Read the model definition and answer for the solid it produces. Units are mm, in the model's axes. A direction names the side the tool comes from. Round coordinates to 2 decimals unless told otherwise and drop trailing zeros. Order: outer loops, then holes, each group sorted by start corner. A loop starts at its lowest first (then second) coordinate and runs counter-clockwise, first axis right, second up. Notation, with made-up numbers: (85, -22.5) - (95, -22.5) arc R25 cw to (95, 12.5) - close; hole circle Ø6 at (4, 31). An arc over 180 degrees is marked (long way). Answer as a JSON object with one key per item and string values. Group by question number.
Q1. Given pin 1 Ø6.5 at (x, y) = (-17.5, 6.12) entering from -Z; pin 2 Ø1.5 at (y, z) = (2, 8.5) entering from -X; pin 3 Ø10 at (x, z) = (3.5, 21.5) entering from +Y, each flat-ended and moving along its own axis, determine where each tip first touches the part or whether it passes through.
Q2. A tool of negligible diameter and unlimited length cuts with its end or side. For faces 4 (the flat face through (-20.5, 9.2, 6)), 5 (the cylindrical face through (-9.34, 0.51, 4.31)), 6 (the cylindrical face through (-20.674, 3.689, -0.084)), from which of +Z, -Z, +X, -X, +Y, -Y can it reach the whole face along a straight path? Write none if from no direction.
Q3. A cutting plane is placed at D-D on z = 23.5. Determine the outline of the cut face in (x, y).
Q4. A cutting plane is placed at B-B on y = 4. Determine the outline of the cut face in (x, z), and give its area (3 significant figures).
Q5. Consider line 1 (Z direction, x = -7.5, y = 0.2); line 2 (Z direction, x = 7.5, y = 0.35); line 3 (Y direction, x = 8, z = -10). Determine where each line is inside the solid, lowest interval first.
Q6. A cutting plane is placed at A-A on x = -17.5. Determine the outline of the cut face in (y, z).
Q7. The mould has two halves that part along Y. Classify faces 1 (the flat face through (-14, 5, 30)), 2 (the flat face through (-18, 0, 0)), 3 (the cylindrical face through (-20.674, 3.689, -24.084)): pulls with the +Y half, pulls with the -Y half, needs draft (parallel to the pull), parting line crosses it, or undercut.
Q8. A cutting plane is placed at C-C on x = 7.5. Determine the outline of the cut face in (y, z), and give its area (3 significant figures).
```python
from build123d import *

# Parameters (mm, degrees)
SKETCH1_W           = 30
SKETCH1_H           = 60
BOSS_EXTRUDE1_DEPTH = 3
SKETCH2_R           = 4
BOSS_EXTRUDE2_DEPTH = 12
SKETCH3_R           = 4
BOSS_EXTRUDE3_DEPTH = 6
SKETCH8_R           = 2.5
CUT_EXTRUDE1_DEPTH  = 4
CHAMFER1_SIZE       = 1
CHAMFER1_SIZE2      = 2
SKETCH9_R           = 4
BOSS_EXTRUDE4_DEPTH = 2


with BuildPart() as part:
    # Sketch1 → Boss-Extrude1 (new body)
    with BuildSketch(Plane(origin=(0, 0, 0), x_dir=(1, 0, 0), z_dir=(0, 1, 0))):
        Rectangle(SKETCH1_W, SKETCH1_H)
    extrude(amount=BOSS_EXTRUDE1_DEPTH)

    # Sketch2 → Boss-Extrude2 (add)
    with BuildSketch(Plane.XY.offset(30)):
        with BuildLine():
            Line((-15, 0), (-20, 0))
            ThreePointArc((-20, 0), (-17.5, 12.735742832), (-15, 0))
        make_face()
        with Locations((-17.5, 6.122498999)):
            Circle(SKETCH2_R, mode=Mode.SUBTRACT)
    boss_extrude2 = extrude(amount=-BOSS_EXTRUDE2_DEPTH)

    # Mirror1: Boss-Extrude2 across plane
    add(boss_extrude2.mirror(Plane.XY))

    # Sketch3 → Boss-Extrude3 (add, symmetric)
    with BuildSketch(Plane.XY):
        with BuildLine():
            Line((-19.72149558, 0), (-15.27850442, 0))
            ThreePointArc((-15.27850442, 0), (-17.5, 12.635565605), (-19.72149558, 0))
        make_face()
        with Locations((-17.5, 6.122498999)):
            Circle(SKETCH3_R, mode=Mode.SUBTRACT)
    extrude(amount=BOSS_EXTRUDE3_DEPTH, both=True)

    # Sketch8 → Cut-Extrude1 (cut, through all)
    with BuildSketch(Plane(origin=(0, 3, 0), x_dir=(1, 0, 0), z_dir=(0, 1, 0))):
        with Locations((7.5, -18)):
            Circle(SKETCH8_R)
        with Locations((-7.5, -6)):
            Circle(SKETCH8_R)
        with Locations((7.5, 6)):
            Circle(SKETCH8_R)
        with Locations((-7.5, 18)):
            Circle(SKETCH8_R)
    extrude(amount=-CUT_EXTRUDE1_DEPTH, mode=Mode.SUBTRACT)

    # Chamfer1
    chamfer1_edges = [part.edges().sort_by_distance(p)[0] for p in [
        (-10, 3, -18),
        (-10, 3, 6),
        (5, 3, 18),
        (5, 3, -6),
    ]]
    chamfer1_side = [part.faces().sort_by_distance(p)[0] for p in [
        (0.987193721, 3, 0),
    ]]
    chamfer(chamfer1_edges, length=CHAMFER1_SIZE, length2=CHAMFER1_SIZE2, reference=chamfer1_side[0])

    # Sketch9 → Boss-Extrude4 (add)
    with BuildSketch(Plane.XY.offset(30)):
        with Locations((-17.5, 6.122498999)):
            Circle(SKETCH9_R)
    extrude(amount=-BOSS_EXTRUDE4_DEPTH)


solid = part.part
```
Result set:
{
 "1": {"pin 1": "stops at z = 28", "pin 2": "stops at x = -15", "pin 3": "stops at y = 3"},
 "2": {"face 4": "-X, +Y", "face 5": "+Y, -Y", "face 6": "-Z"},
 "3": {"outline": "(-20, 0) - (15, 0) - (15, 3) - (-11.67, 3) arc R6.61 ccw (long way) to start; hole circle Ø8 at (-17.5, 6.12)"},
 "4": {"outline": "(-23.76, -30) - (-20.89, -30) - (-20.89, -18) - (-23.76, -18) - close; (-23.76, 18) - (-20.89, 18) - (-20.89, 28) - (-14.11, 28) - (-14.11, 18) - (-11.24, 18) - (-11.24, 30) - (-23.76, 30) - close; (-23.66, -6) - (-20.89, -6) - (-20.89, 6) - (-23.66, 6) - close; (-14.11, -30) - (-11.24, -30) - (-11.24, -18) - (-14.11, -18) - close; (-14.11, -6) - (-11.34, -6) - (-11.34, 6) - (-14.11, 6) - close", "area": "218 mm²"},
 "5": {"line 1": "z = -30 to -20.5, -15.5 to 3.5, 8.5 to 30", "line 2": "z = -30 to -8.5, -3.5 to 15.5, 20.5 to 30", "line 3": "y = 0 to 3"},
 "6": {"outline": "(0, -30) - (2.12, -30) - (2.12, -18) - (0, -18) - close; (0, -6) - (2.12, -6) - (2.12, 6) - (0, 6) - close; (0, 18) - (2.12, 18) - (2.12, 28) - (10.12, 28) - (10.12, 18) - (12.74, 18) - (12.74, 30) - (0, 30) - close; (10.12, -30) - (12.74, -30) - (12.74, -18) - (10.12, -18) - close; (10.12, -6) - (12.64, -6) - (12.64, 6) - (10.12, 6) - close"},
 "7": {"face 1": "needs draft", "face 2": "pulls with the -Y half", "face 3": "undercut"},
 "8": {"outline": "(0, -30) - (3, -30) - (3, -9.5) - (1, -8.5) - (0, -8.5) - close; (0, -3.5) - (1, -3.5) - (3, -2.5) - (3, 14.5) - (1, 15.5) - (0, 15.5) - close; (0, 20.5) - (1, 20.5) - (3, 21.5) - (3, 30) - (0, 30) - close", "area": "146 mm²"}
}
